from build123d import *

# Parameters (mm, degrees)
SKETCH2_W                         = 218.44
SKETCH2_H                         = 50.8
SKETCH2_R                         = 3.81
BOSS_EXTRUDE1_DEPTH               = 2.54
SKETCH3_W                         = 182.88
SKETCH3_H                         = 40.64
BOSS_EXTRUDE2_DEPTH               = 101.6
SKETCH5_W                         = 137.16
SKETCH5_H                         = 76.2
CUT_EXTRUDE2_DEPTH                = 101.6
FILLET1_R                         = 17.78
FILLET2_R                         = 17.78
FILLET3_R                         = 12.7
FILLET4_R                         = 12.7
FILLET5_R                         = 2.54
FILLET6_R                         = 2.54
N_0_302_DIAMETER_HOLE1_AT_2_COUNT = 2
N_0_302_DIAMETER_HOLE1_AT_2_PITCH = 203.2


with BuildPart() as part:
    # Sketch2 → Boss-Extrude1 (new body)
    with BuildSketch(Plane(origin=(0, 0, 0), x_dir=(1, 0, 0), z_dir=(0, 1, 0))):
        with Locations((109.22, 25.4)):
            Rectangle(SKETCH2_W, SKETCH2_H)
        with Locations(Location((7.62, 25.4, 0), (0, 0, 270))):
            Circle(SKETCH2_R, mode=Mode.SUBTRACT)
        with Locations(Location((210.82, 25.4, 0), (0, 0, 90))):
            Circle(SKETCH2_R, mode=Mode.SUBTRACT)
    extrude(amount=BOSS_EXTRUDE1_DEPTH)

    # Sketch3 → Boss-Extrude2 (add)
    with BuildSketch(Plane(origin=(0, 2.54, 0), x_dir=(1, 0, 0), z_dir=(0, 1, 0))):
        with Locations((109.22, 25.4)):
            Rectangle(SKETCH3_W, SKETCH3_H)
    extrude(amount=BOSS_EXTRUDE2_DEPTH)

    # Sketch5 → Cut-Extrude2 (cut)
    with BuildSketch(Plane.XY.offset(-5.08)):
        with Locations((109.22, 40.64)):
            Rectangle(SKETCH5_W, SKETCH5_H)
    extrude(amount=-CUT_EXTRUDE2_DEPTH, mode=Mode.SUBTRACT)

    # Fillet1
    fillet1_edges = [part.edges().sort_by_distance(p)[0] for p in [
        (109.22, 104.14, -5.08),
    ]]
    fillet(fillet1_edges, radius=FILLET1_R)

    # Fillet2
    fillet2_edges = [part.edges().sort_by_distance(p)[0] for p in [
        (109.22, 104.14, -45.72),
    ]]
    fillet(fillet2_edges, radius=FILLET2_R)

    # Fillet3
    fillet3_edges = [part.edges().sort_by_distance(p)[0] for p in [
        (17.78, 44.45, -5.08),
        (17.78, 98.932358569, -10.287641431),
        (17.78, 104.14, -25.4),
        (17.78, 44.45, -45.72),
        (17.78, 98.932358569, -40.512358569),
    ]]
    fillet(fillet3_edges, radius=FILLET3_R)

    # Fillet4
    fillet4_edges = [part.edges().sort_by_distance(p)[0] for p in [
        (200.66, 104.14, -25.4),
        (200.66, 44.45, -5.08),
        (200.66, 98.932358569, -10.287641431),
        (200.66, 44.45, -45.72),
        (200.66, 98.932358569, -40.512358569),
    ]]
    fillet(fillet4_edges, radius=FILLET4_R)

    # Fillet5
    fillet5_edges = [part.edges().sort_by_distance(p)[0] for p in [
        (40.64, 2.54, -25.4),
    ]]
    fillet(fillet5_edges, radius=FILLET5_R)

    # Fillet6
    fillet6_edges = [part.edges().sort_by_distance(p)[0] for p in [
        (177.8, 2.54, -25.4),
    ]]
    fillet(fillet6_edges, radius=FILLET6_R)

    # Sketch7 → N (0.302) Diameter Hole1 (revolve, cut)
    with BuildSketch(Plane(origin=(210.82, 2.54, -25.4), x_dir=(0, 0, 1), z_dir=(1, 0, 0))):
        Polygon((0, 0), (0, 2.54), (3.8354, 2.54), (3.8354, 0.532828266), (4.4704, 0), align=None)
    n_0_302_diameter_hole1 = revolve(axis=Axis((210.82, 8.89, -25.4), (0, -1, 0)), mode=Mode.SUBTRACT)

    # N (0.302) Diameter Hole1 at 2: N (0.302) Diameter Hole1 ×2
    with Locations(*[(-i * N_0_302_DIAMETER_HOLE1_AT_2_PITCH, 0, 0) for i in range(1, N_0_302_DIAMETER_HOLE1_AT_2_COUNT)]):
        add(n_0_302_diameter_hole1, mode=Mode.SUBTRACT)


solid = part.part
CAD build for the part. Positions are in the model's coordinates, mm. A direction names the side the tool comes from. Give positions to 0.01 mm unless a question says otherwise; leave off trailing zeros. Order: outer loops, then holes, each group sorted by start corner. A loop starts at its lowest first (then second) coordinate and runs counter-clockwise, first axis right, second up. Notation, with made-up numbers: (42, 35) -> (86, 35) arc R32 ccw to (86, 71) -> close; hole circle Ø7 at (24.5, 61). An arc over 180 degrees is marked (long way). Return JSON: item names as keys, results as strings.
Q1. Flat gauge pins, fed straight in: pin 1 (20.5 mm diameter, centred on y = 34.5, z = -16.5, fed in from -X); pin 2 (8 mm diameter, centred on y = 28, z = -45, fed in from +X); pin 3 (6 mm diameter, centred on x = 70.5, y = 80.5, fed in from +Z); pin 4 (7 mm diameter, centred on x = 7.62, z = -25.4, fed in from +Y). Where does each tip first touch, or does it go through?
Working result:
{"pin 1": "x = 17.78", "pin 2": "x = 197.84", "pin 3": "z = -5.08", "pin 4": "through"}
Q2. Saw through at B-B (z = -25.4). Write the cut outline in (x, y), then the cut area to 3 significant figures.
Working result:
{"outline": "(0, 0) -> (3.78, 0) -> (3.78, 2.01) -> (3.15, 2.54) -> (0, 2.54) -> close; (11.46, 0) -> (206.98, 0) -> (206.98, 2.01) -> (206.35, 2.54) -> (200.66, 2.54) -> (200.66, 91.44) arc R12.7 ccw to (187.96, 104.14) -> (30.48, 104.14) arc R12.7 ccw to (17.78, 91.44) -> (17.78, 2.54) -> (12.09, 2.54) -> (11.46, 2.01) -> close; (214.66, 0) -> (218.44, 0) -> (218.44, 2.54) -> (215.29, 2.54) -> (214.66, 2.01) -> close; hole (40.64, 5.08) arc R2.54 ccw to (43.18, 2.54) -> (175.26, 2.54) arc R2.54 ccw to (177.8, 5.08) -> (177.8, 78.74) -> (40.64, 78.74) -> close", "area": "8,580 mm²"}
Q3. Mould opens along Z. For faces 1 (the face through (110.322, 99.07, -40.373)), 2 (the face through (108, 104.14, -25)), 3 (the face through (5, 1, -28.2)) say: pulls with the +Z half, pulls with the -Z half, needs draft (parallel to the pull), parting line crosses it, or undercut.
Working result:
{"face 1": "pulls with the -Z half", "face 2": "needs draft", "face 3": "undercut"}
Q4. Saw through at D-D (x = 149). Write the cut outline in (y, z), then the cut area to 3 significant figures.
Working result:
{"outline": "(0, -50.8) -> (2.54, -50.8) -> (2.54, 0) -> (0, 0) -> close; (78.74, -45.72) -> (86.36, -45.72) arc R17.78 ccw to (104.14, -27.94) -> (104.14, -22.86) arc R17.78 ccw to (86.36, -5.08) -> (78.74, -5.08) -> close", "area": "1,030 mm²"}
Q5. Drill centre lines: line 1 (X direction, y = 1, z = -25); line 2 (Z direction, x = 210.82, y = 0.55); line 3 (X direction, y = 0.5, z = -25.4). Where is each one in solid material? Low to high.
Working result:
{"line 1": "0 to 3.81, 11.43 to 207.01, 214.63 to 218.44", "line 2": "-50.8 to -29.24, -21.56 to 0", "line 3": "0 to 3.78, 11.46 to 206.98, 214.66 to 218.44"}
Q6. Which spindle directions (+Z, -Z, +X, -X, +Y, -Y) get a long thin tool onto all of the face, cutting with end or side? Do faces 4 (the face through (17.78, 46, -25)), 5 (the face through (21.6, 43.9, -42.1)), 6 (the face through (109, 82, -45.72)). Say none if no direction does.
Working result:
{"face 4": "+Z, -Z, -X, +Y", "face 5": "-Z, -X, +Y", "face 6": "-Z, +X, -X, +Y"}
Q7. Saw through at C-C (x = 7.62). Write the cut outline in (y, z).
Working result:
{"outline": "(0, -50.8) -> (2.54, -50.8) -> (2.54, -29.87) -> (2.01, -29.24) -> (0, -29.24) -> close; (0, -21.56) -> (2.01, -21.56) -> (2.54, -20.93) -> (2.54, 0) -> (0, 0) -> close"}
Q8. Saw through at A-A (y = 70.5). Write the cut outline in (x, z).
Working result:
{"outline": "(17.78, -33.02) arc R12.7 ccw to (30.48, -45.72) -> (40.64, -45.72) -> (40.64, -5.08) -> (30.48, -5.08) arc R12.7 ccw to (17.78, -17.78) -> close; (177.8, -45.72) -> (187.96, -45.72) arc R12.7 ccw to (200.66, -33.02) -> (200.66, -17.78) arc R12.7 ccw to (187.96, -5.08) -> (177.8, -5.08) -> close"}
